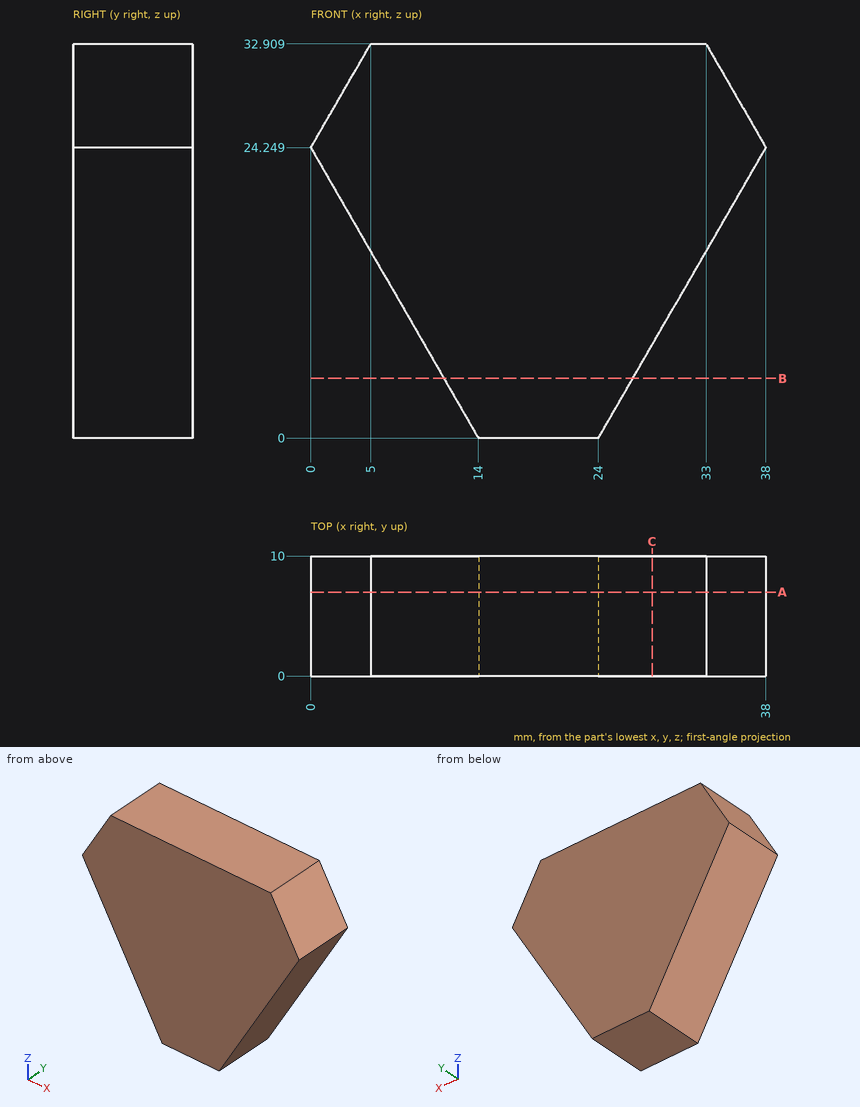
Job drawing, mm, ordinate dimensions from the low corner. One solid piece. Give positions to 0.01 mm unless a question says otherwise; leave off trailing zeros. Write each loop counter-clockwise with the first axis right and the second up, starting at its lowest first coordinate (ties: lowest second). Pieces come first, ordered by that corner, then holes. Notation, with made-up numbers: (88, 22.25) - (134, 22.25) arc R11 cw to (134, 37.25) - close; hole circle Ø3 at (-19.75, -40). An arc over 180 degrees is marked (long way). Use one line per item in the form item = value. Start each with the question number.
1. Drop flat-ended pins along their axis: pin 1 Ø1.5 at (y, z) = (5, 13.5) entering from +X; pin 2 Ø4 at (y, z) = (6, 16) entering from -X; pin 3 Ø1.5 at (y, z) = (7.5, 9.5) entering from +X. Give the stop position or say it passes through.
2. Band-saw the part on B-B on z = 5. Write the cut outline in (x, y).
3. Band-saw the part on C-C on x = 28.5. Write the cut outline in (y, z), plus the area to 3 significant figures.
4. Band-saw the part on A-A on y = 7. Write the cut outline in (x, z).
5. Probe line 1 (X direction, y = 4, z = 5.5) (1 decimal); line 2 (Z direction, x = 9.5, y = 5.75) (1 decimal); line 3 (Z direction, x = 32.5, y = 6.75) (1 decimal). List the from-to ranges inside material, lowest first. Write a range as [from, to].
Conclusion:
q1.pin_1 = 32.23
q1.pin_2 = 3.61
q1.pin_3 = 29.92
q2.outline = (11.11, 0) - (26.89, 0) - (26.89, 10) - (11.11, 10) - close
q3.outline = (0, 7.79) - (10, 7.79) - (10, 32.91) - (0, 32.91) - close
q3.area = 251 mm²
q4.outline = (0, 24.25) - (14, 0) - (24, 0) - (38, 24.25) - (33, 32.91) - (5, 32.91) - close
q5.line_1 = [10.8, 27.2]
q5.line_2 = [7.8, 32.9]
q5.line_3 = [14.7, 32.9]
